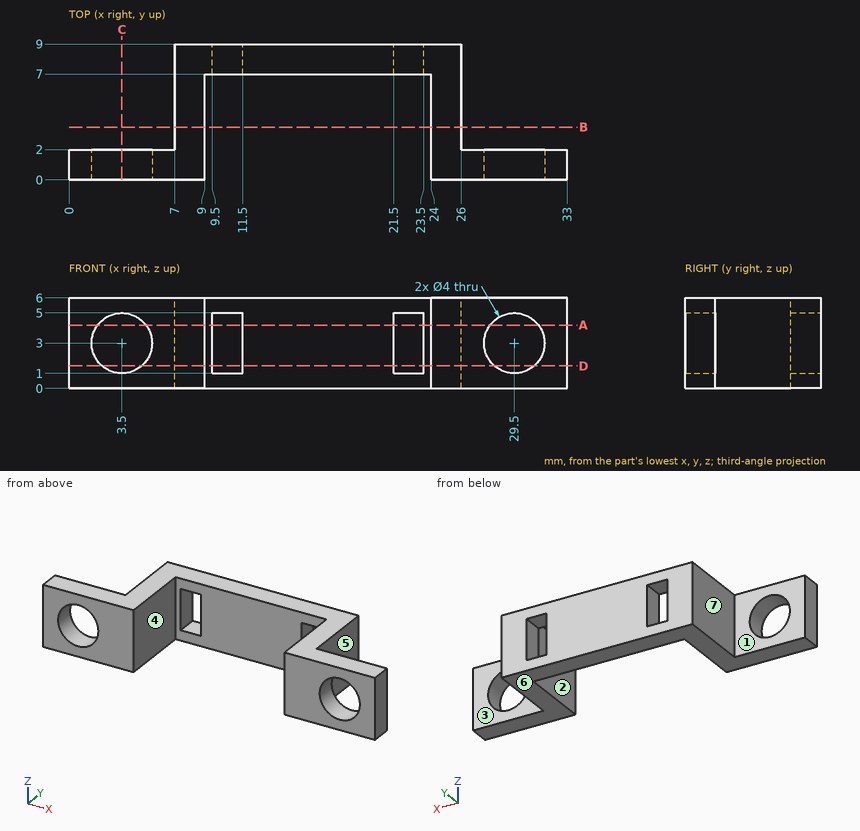
Could you check a few things on this drawing? It's one solid part, dimensions in mm from its lowest x, y, z. A direction names the side the tool comes from. Give positions to 0.01 mm unless a question says otherwise; leave off trailing zeros. Order: outer loops, then holes, each group sorted by start corner. A loop starts at its lowest first (then second) coordinate and runs counter-clockwise, first axis right, second up. Notation, with made-up numbers: (-24, 77.5) -> (34, 77.5) arc R19 ccw to (34, 94.5) -> close; hole circle Ø10 at (-15.75, -8.75). An arc over 180 degrees is marked (long way). Use CSV: the item, a comma, the result in double quotes. Start each with the question number.
Item 1: Thinking about a two-plate mould opening in X: for the marked faces 4, 5, 6 and 7, which applies, pulls with the +X half, pulls with the -X half, needs draft (parallel to the pull), parting line crosses it, or undercut?
Item 2: Suppose I cut it at C-C (x = 3.5). List the corners of the cut face in (y, z) for me.
Item 3: Suppose I cut it at B-B (y = 3.5). List the corners of the cut face in (x, z) for me, and give its area (3 significant figures).
Item 4: Suppose I cut it at D-D (z = 1.5). List the corners of the cut face in (x, y) for me.
Item 5: If I drill on probe 1 along X at (y, z) = (0.8, 3); probe 2 along X at (y, z) = (3, 5.1); probe 3 along Z at (x, y) = (3.5, 1.3), over which ranges is the centre line in solid material (lowest first)? Write a range as [from, to].
Item 6: Suppose I cut it at A-A (z = 4.2). List the corners of the cut face in (x, y) for me, and give its area (3 significant figures).
Item 7: I'm going to push flat-ended pins straight in: P1, Ø1.8, axis at x = 16.5, z = 1.5, coming from the -Y side; P2, Ø3, axis at x = 5, z = 3.5, coming from the +Y side; P3, Ø1.6, axis at y = 7.5, z = 2.5, coming from the +X side. Where does each tip first touch, or does it pass through?
Item 8: On a 3-axis mill with a long thin cutter (end or side, diameter ignored), from which of +Z, -Z, +X, -X, +Y, -Y can I reach the whole of each face in a straight line? I mean the marked faces 1, 2 and 3. Say none if no direction works.
Answer block:
1,face 4,"undercut"
1,face 5,"pulls with the +X half"
1,face 6,"needs draft"
1,face 7,"pulls with the -X half"
2,outline,"(0, 0) -> (2, 0) -> (2, 1) -> (0, 1) -> close; (0, 5) -> (2, 5) -> (2, 6) -> (0, 6) -> close"
3,outline,"(7, 0) -> (9, 0) -> (9, 6) -> (7, 6) -> close; (24, 0) -> (26, 0) -> (26, 6) -> (24, 6) -> close"
3,area,"24.0 mm^2"
4,outline,"(0, 0) -> (2.18, 0) -> (2.18, 2) -> (0, 2) -> close; (4.82, 0) -> (9, 0) -> (9, 7) -> (9.5, 7) -> (9.5, 9) -> (7, 9) -> (7, 2) -> (4.82, 2) -> close; (11.5, 7) -> (21.5, 7) -> (21.5, 9) -> (11.5, 9) -> close; (23.5, 7) -> (24, 7) -> (24, 0) -> (28.18, 0) -> (28.18, 2) -> (26, 2) -> (26, 9) -> (23.5, 9) -> close; (30.82, 0) -> (33, 0) -> (33, 2) -> (30.82, 2) -> close"
5,probe 1,"x = [0, 1.5], [5.5, 9], [24, 27.5], [31.5, 33]"
5,probe 2,"x = [7, 9], [24, 26]"
5,probe 3,"z = [0, 1], [5, 6]"
6,outline,"(0, 0) -> (1.9, 0) -> (1.9, 2) -> (0, 2) -> close; (5.1, 0) -> (9, 0) -> (9, 7) -> (9.5, 7) -> (9.5, 9) -> (7, 9) -> (7, 2) -> (5.1, 2) -> close; (11.5, 7) -> (21.5, 7) -> (21.5, 9) -> (11.5, 9) -> close; (23.5, 7) -> (24, 7) -> (24, 0) -> (27.9, 0) -> (27.9, 2) -> (26, 2) -> (26, 9) -> (23.5, 9) -> close; (31.1, 0) -> (33, 0) -> (33, 2) -> (31.1, 2) -> close"
6,area,"73.2 mm^2"
7,P1,"stops at y = 7"
7,P2,"stops at y = 2"
7,P3,"stops at x = 26"
8,face 1,"+Z, -Z, -X, +Y"
8,face 2,"+Z, -Z, -Y"
8,face 3,"+Z, -Z, +X, +Y"
